from build123d import *

# Parameters (mm, degrees)
SKETCH_1_R          = 14.975
EXTRUDE_1_DEPTH     = 9
SKETCH_2_R          = 1.65
CUT_EXTRUDE_1_DEPTH = 10
SKETCH_3_R          = 2.1
CUT_EXTRUDE_2_DEPTH = 24.010894159
SKETCH_4_R          = 3.65
CUT_EXTRUDE_3_DEPTH = 4


with BuildPart() as part:
    # 草图1 → 凸台-拉伸1 (new body)
    with BuildSketch(Plane(origin=(0, 0, 0), x_dir=(1, 0, 0), z_dir=(0, 1, 0))):
        with Locations(Location((0, 0, 0), (0, 0, 270))):
            Circle(SKETCH_1_R)
    extrude(amount=EXTRUDE_1_DEPTH)

    # 草图2 → 切除-拉伸1 (cut)
    with BuildSketch(Plane.XZ):
        with Locations(Location((-11, 0, 0), (0, 0, 270))):
            Circle(SKETCH_2_R)
        with Locations(Location((-5.5, 9.526279442, 0), (0, 0, 270))):
            Circle(SKETCH_2_R)
        with Locations(Location((5.5, 9.526279442, 0), (0, 0, 270))):
            Circle(SKETCH_2_R)
        with Locations(Location((11, 0, 0), (0, 0, 270))):
            Circle(SKETCH_2_R)
        with Locations(Location((5.5, -9.526279442, 0), (0, 0, 270))):
            Circle(SKETCH_2_R)
        with Locations(Location((-5.5, -9.526279442, 0), (0, 0, 270))):
            Circle(SKETCH_2_R)
    extrude(amount=-CUT_EXTRUDE_1_DEPTH, mode=Mode.SUBTRACT)

    # 草图3 → 切除-拉伸2 (cut, through all)
    with BuildSketch(Plane.XZ):
        with Locations(Location((0, 5, 0), (0, 0, 270))):
            Circle(SKETCH_3_R)
        with Locations(Location((4.330127019, -2.5, 0), (0, 0, 270))):
            Circle(SKETCH_3_R)
        with Locations(Location((-4.330127019, -2.5, 0), (0, 0, 270))):
            Circle(SKETCH_3_R)
    extrude(amount=-CUT_EXTRUDE_2_DEPTH, mode=Mode.SUBTRACT)

    # 草图4 → 切除-拉伸3 (cut)
    with BuildSketch(Plane.XZ):
        with Locations(Location((0, 5, 0), (0, 0, 270))):
            Circle(SKETCH_4_R)
        with Locations(Location((-4.330127019, -2.5, 0), (0, 0, 270))):
            Circle(SKETCH_4_R)
        with Locations(Location((4.330127019, -2.5, 0), (0, 0, 270))):
            Circle(SKETCH_4_R)
    extrude(amount=-CUT_EXTRUDE_3_DEPTH, mode=Mode.SUBTRACT)


solid = part.part
Check sheet for the modelled part. Datum: model origin and axes. Units: mm. A direction names the side the tool comes from. Round coordinates to 2 decimals unless told otherwise and drop trailing zeros. Order: outer loops, then holes, each group sorted by start corner. A loop starts at its lowest first (then second) coordinate and runs counter-clockwise, first axis right, second up.
(1) Cross-section at D-D, the plane y = 1.5. State how many separate pieces and enclosed holes the cut face has, and give its area (3 significant figures).
(2) Go/stop test with flat-tipped pins: P1, Ø4, axis at x = 3, y = 3, coming from the +Z side; P2, Ø4, axis at y = 2, z = -4, coming from the -X side; P3, Ø3.5, axis at x = 0.5, z = 4.5, coming from the -Y side. Record where each tip stops, or that it passes through.
(3) Cross-section at A-A, the plane x = 0. Enter the section's corners in (y, z) (3 decimals), and give its area (3 significant figures).
(4) Access from +Z, -Z, +X, -X, +Y, -Y to the whole of each face (thin tool, end or side, straight path). Record for faces 4 (the cylindrical face through (-5.427, 4.437, 11.175)), 5 (the cylindrical face through (1.1, 1.97, 1.52)).
(5) Scan lines: probe 1 along Z at (x, y) = (6, 6.5); probe 2 along Z at (x, y) = (-2.5, 0.5); probe 3 along X at (y, z) = (3.75, -9.5). Record each from-to range of solid material in increasing order.
(6) Cross-section at C-C, the plane z = 6.5. Enter the section's corners in (x, y), and give its area (3 significant figures).
(7) Cross-section at B-B, the plane z = -2.5. Enter the section's corners in (x, y).
(8) Draft check along X on faces 1 (the flat face through (0, 9, 0)), 2 (the cylindrical face through (2.28, 6.46, -2.04)), 3 (the cylindrical face through (14.848, 4.437, -1.949)). Enter one of: pulls with the +X half, pulls with the -X half, needs draft (parallel to the pull), parting line crosses it, or undercut.
Check sheet entries:
1. separate pieces: 1
1. enclosed holes: 9
1. area: 528 mm2
2. P1: stops at z = 14.94
2. P2: stops at x = -14.84
2. P3: stops at y = 4
3. outline: (0, -14.975) - (9, -14.975) - (9, 2.9) - (4, 2.9) - (4, 1.35) - (0, 1.35) - close; (0, 8.65) - (4, 8.65) - (4, 7.1) - (9, 7.1) - (9, 14.975) - (0, 14.975) - close
3. area: 219 mm2
4. face 4: +Y, -Y
4. face 5: -Y
5. probe 1: z = -13.72 to -11.1, -7.95 to -3.77, -1.23 to 7.95, 11.1 to 13.72
5. probe 2: z = -14.76 to -5.66, 0.66 to 2.34, 7.66 to 14.76
5. probe 3: x = -11.58 to -7.15, -3.85 to 3.85, 7.15 to 11.58
6. outline: (-13.49, 0) - (-3.33, 0) - (-3.33, 4) - (-1.47, 4) - (-1.47, 9) - (-13.49, 9) - close; (1.47, 4) - (3.33, 4) - (3.33, 0) - (13.49, 0) - (13.49, 9) - (1.47, 9) - close
6. area: 202 mm2
7. outline: (-14.76, 0) - (-7.98, 0) - (-7.98, 4) - (-6.43, 4) - (-6.43, 9) - (-14.76, 9) - close; (-2.23, 4) - (-0.68, 4) - (-0.68, 0) - (0.68, 0) - (0.68, 4) - (2.23, 4) - (2.23, 9) - (-2.23, 9) - close; (6.43, 4) - (7.98, 4) - (7.98, 0) - (14.76, 0) - (14.76, 9) - (6.43, 9) - close
8. face 1: needs draft
8. face 2: undercut
8. face 3: parting line crosses it
